```python
from build123d import *

# Parameters (mm, degrees)
SKETCH1_W           = 40
SKETCH1_H           = 12
BOSS_EXTRUDE1_DEPTH = 3
SKETCH3_R           = 1.25
CUT_EXTRUDE2_DEPTH  = 22.09502311
CUT_EXTRUDE3_DEPTH  = 10
FILLET2_R           = 5
FILLET3_R           = 1
FILLET4_R           = 5
FILLET5_R           = 5


with BuildPart() as part:
    # Sketch1 → Boss-Extrude1 (new body)
    with BuildSketch(Plane(origin=(0, 0, 0), x_dir=(1, 0, 0), z_dir=(0, 1, 0))):
        Rectangle(SKETCH1_W, SKETCH1_H)
    extrude(amount=BOSS_EXTRUDE1_DEPTH)

    # Sketch3 → Cut-Extrude2 (cut, through all)
    with BuildSketch(Plane(origin=(0, 3, 0), x_dir=(1, 0, 0), z_dir=(0, 1, 0))):
        with Locations(Location((-17.5, 3.5, 0), (0, 0, 270))):
            Circle(SKETCH3_R)
        with Locations(Location((-17.5, -3.5, 0), (0, 0, 270))):
            Circle(SKETCH3_R)
    extrude(amount=-CUT_EXTRUDE2_DEPTH, mode=Mode.SUBTRACT)

    # Sketch5 → Cut-Extrude3 (cut)
    with BuildSketch(Plane(origin=(0, 3, 0), x_dir=(1, 0, 0), z_dir=(0, 1, 0))):
        with BuildLine():
            Line((-13.458222524, 6), (20, 0))
            Line((20, 0), (20, -6))
            Line((20, -6), (17.030073052, -6))
            ThreePointArc((17.030073052, -6), (7.671541519, -2.617819669), (-2.144608615, -4.250134828))
            Line((-2.144608615, -4.250134828), (-6.569653649, -6))
            Line((-6.569653649, -6), (-13.458222524, -6))
            Line((-13.458222524, -6), (-13.458222524, -10.237178745))
            Line((-13.458222524, -10.237178745), (26.023482417, -9.726914384))
            Line((26.023482417, -9.726914384), (26.023482417, 8.477274399))
            Line((26.023482417, 8.477274399), (-13.458222524, 8.477274399))
            Line((-13.458222524, 8.477274399), (-13.458222524, 6))
        make_face()
    extrude(amount=-CUT_EXTRUDE3_DEPTH, mode=Mode.SUBTRACT)

    # Fillet2
    # the kernel refuses this fillet: 5 mm, written as the material it takes off along each edge
    with BuildSketch(Plane(origin=(-6.569653649, 5.381801612, 6), x_dir=(-1, 0, 0), z_dir=(0, -1, 0))) as fillet2_piece_1:
        with BuildLine():
            CenterArc((FILLET2_R * 0.190544128998, FILLET2_R), FILLET2_R, 248.423891744, 21.576108256)
            Line((-FILLET2_R * 0.17719268457, FILLET2_R * 0.0700700908417), (0, 0))
            Line((0, 0), (FILLET2_R * 0.190544128998, 0))
        make_face()
    extrude(amount=7.763603225, mode=Mode.SUBTRACT)
    with BuildSketch(Plane(origin=(-2.144608615, 3.259446384, 4.250134828), x_dir=(-0.9299299091583175, 0, 0.36773681356753396), z_dir=(0, -1, 0))) as fillet2_piece_2:
        with BuildLine():
            CenterArc((0.103778554, 5), FILLET2_R, 267.749266862, 2.250733138)
            ThreePointArc((-0.092584454, 0.003857331), (-0.046289955, 0.001983199), (0, 0))
            Line((0, 0), (0.103778554, 0))
        make_face()
    extrude(amount=3.518892769, mode=Mode.SUBTRACT)
    with BuildSketch(Plane(origin=(17.030073052, 6.64587884, 6), x_dir=(1, 0, 0), z_dir=(0, -1, 0))) as fillet2_piece_3:
        with BuildLine():
            CenterArc((1.458351536, -5), FILLET2_R, 90, 30.730822568)
            ThreePointArc((-1.096675494, -0.70211251), (-0.542524687, -0.360136055), (0, 0))
            Line((0, 0), (1.458351536, 0))
        make_face()
    extrude(amount=10.291757681, mode=Mode.SUBTRACT)

    # Fillet3
    fillet3_edges = [part.edges().sort_by_distance(p)[0] for p in [
        (20, 1.5, 6),
    ]]
    fillet(fillet3_edges, radius=FILLET3_R)

    # Fillet4
    fillet4_edges = [part.edges().sort_by_distance(p)[0] for p in [
        (20, 1.5, 0),
    ]]
    fillet(fillet4_edges, radius=FILLET4_R)

    # Fillet5
    fillet5_edges = [part.edges().sort_by_distance(p)[0] for p in [
        (-13.458222524, 1.5, -6),
    ]]
    fillet(fillet5_edges, radius=FILLET5_R)


solid = part.part
```
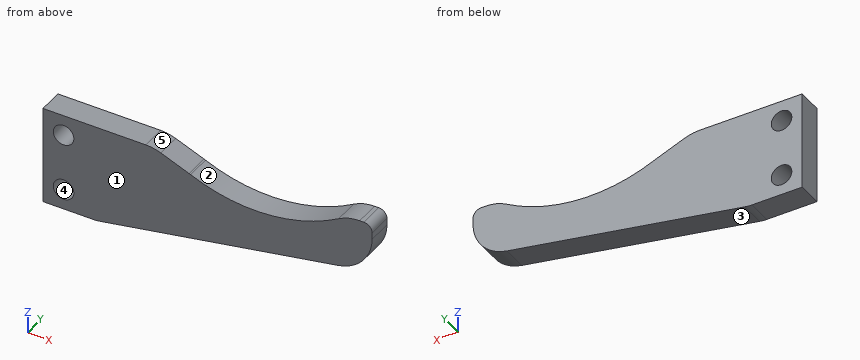
Build history of the part. All positions in model axes, mm. Face numbers are marked on the shaded views. A direction names the side the tool comes from. Round coordinates to 2 decimals unless told otherwise and drop trailing zeros. Write each loop counter-clockwise with the first axis right and the second up, starting at its lowest first coordinate (ties: lowest second). Pieces come first, ordered by that corner, then holes.
1) Mould opens along X. For the marked faces 1, 2 and 3 say: +X half, -X half, draft (parallel to the pull), parting line (faces both ways), or undercut.
2) Band-saw the part on A-A, the plane x = -17.5. List the corners of the cut face in (y, z), and give its area (3 significant figures).
3) Pin check, flat tips, straight feed: pin 1 (2 mm diameter, centred on x = -17.5, z = 3.5, fed in from +Y); pin 2 (1.5 mm diameter, centred on y = 0.5, z = -1, fed in from +X). Stop position of each tip, or through.
4) Band-saw the part on B-B, the plane y = 0.35. List the corners of the cut face in (x, z), and give its area (3 significant figures).
5) Band-saw the part on D-D, the plane z = 3.5. List the corners of the cut face in (x, y), and give its area (3 significant figures).
6) Band-saw the part on C-C, the plane z = -3.5. List the corners of the cut face in (x, y), and give its area (3 significant figures).
7) 3-axis set-ups, long thin cutter, end or side, ignore diameter. For the marked faces 4 and 5: which of +Z, -Z, +X, -X, +Y, -Y reach the whole face in a straight line?
8) Drill centre lines: probe 1 along X at (y, z) = (1.3, 0.5); probe 2 along Z at (x, y) = (9, 0.2); probe 3 along Z at (x, y) = (1.5, 1.85). Where is each one in solid material? Low to high.
Ans:
1. face 1: draft
1. face 2: undercut
1. face 3: +X half
2. outline: (0, -6) - (3, -6) - (3, -4.75) - (0, -4.75) - close; (0, -2.25) - (3, -2.25) - (3, 2.25) - (0, 2.25) - close; (0, 4.75) - (3, 4.75) - (3, 6) - (0, 6) - close
2. area: 21.0 mm2
3. pin 1: passes through
3. pin 2: stops at x = 17.31
4. outline: (-20, -6) - (-13.9, -6) arc R5 ccw to (-13.02, -5.92) - (15.88, -0.74) arc R5 ccw to (20, 4.18) - (20, 5) arc R1 ccw to (19, 6) - (18.49, 6) arc R5 ccw to (15.93, 5.3) arc R19.67 cw to (-2.06, 4.21) arc R5 ccw to (-2.24, 4.29) - (-5.68, 5.65) arc R5 ccw to (-7.52, 6) - (-20, 6) - close; hole circle Ø2.5 at (-17.5, -3.5); hole circle Ø2.5 at (-17.5, 3.5)
4. area: 312 mm2
5. outline: (-20, 0) - (-18.75, 0) - (-18.75, 3) - (-20, 3) - close; (-16.25, 0) - (-0.2, 0) - (-0.2, 3) - (-16.25, 3) - close; (11.96, 0) - (19.95, 0) - (19.95, 3) - (11.96, 3) - close
5. area: 75.9 mm2
6. outline: (-20, 0) - (-18.75, 0) - (-18.75, 3) - (-20, 3) - close; (-16.25, 0) - (0.48, 0) - (0.48, 3) - (-16.25, 3) - close
6. area: 53.9 mm2
7. face 4: +Y, -Y
7. face 5: +Z, +Y, -Y
8. probe 1: x = -20 to 18.38
8. probe 2: z = -1.97 to 2.78
8. probe 3: z = -3.32 to 3.03
